```python
from build123d import *

# Parameters (mm, degrees)
SKETCH1_W           = 196.85
SKETCH1_H           = 19.05
SKETCH1_R           = 2.032
BOSS_EXTRUDE1_DEPTH = 3.175
CHAMFER1_SIZE       = 12.7
FILLET1_R           = 5.08
FILLET2_R           = 2.54
CUT_EXTRUDE1_REACH  = 100.936
FILLET3_R           = 3.175
FILLET4_R           = 0.635
FILLET5_R           = 25.4


with BuildPart() as part:
    # Sketch1 → Boss-Extrude1 (new body)
    with BuildSketch(Plane.XY):
        Rectangle(SKETCH1_W, SKETCH1_H)
        with Locations((-73.66, -5.715)):
            Circle(SKETCH1_R, mode=Mode.SUBTRACT)
        with Locations((-85.09, -5.715)):
            Circle(SKETCH1_R, mode=Mode.SUBTRACT)
        with Locations((73.66, -5.715)):
            Circle(SKETCH1_R, mode=Mode.SUBTRACT)
        with Locations((85.09, -5.715)):
            Circle(SKETCH1_R, mode=Mode.SUBTRACT)
    extrude(amount=BOSS_EXTRUDE1_DEPTH)

    # Chamfer1
    chamfer1_edges = [part.edges().sort_by_distance(p)[0] for p in [
        (-98.425, 9.525, 1.5875),
        (98.425, 9.525, 1.5875),
    ]]
    chamfer(chamfer1_edges, length=CHAMFER1_SIZE)

    # Fillet1
    fillet1_edges = [part.edges().sort_by_distance(p)[0] for p in [
        (-85.725, 9.525, 1.5875),
        (85.725, 9.525, 1.5875),
        (98.425, -3.175, 1.5875),
        (-98.425, -3.175, 1.5875),
    ]]
    fillet(fillet1_edges, radius=FILLET1_R)

    # Fillet2
    fillet2_edges = [part.edges().sort_by_distance(p)[0] for p in [
        (98.425, -9.525, 1.5875),
        (-98.425, -9.525, 1.5875),
    ]]
    fillet(fillet2_edges, radius=FILLET2_R)

    # Sketch2 → Cut-Extrude1 (cut, up to next)
    with BuildSketch(Plane.XY.offset(3.175), mode=Mode.PRIVATE) as cut_extrude1_sk1:
        Polygon((-62.264047257, 5.715), (-36.195, 1.288180654), (-10.125952743, 5.715), align=None)
    cut_extrude1_tool1 = extrude(cut_extrude1_sk1.sketch, amount=-CUT_EXTRUDE1_REACH, mode=Mode.PRIVATE) & part.part
    # Sketch2 → Cut-Extrude1 (cut, up to next)
    with BuildSketch(Plane.XY.offset(3.175), mode=Mode.PRIVATE) as cut_extrude1_sk2:
        Polygon((-69.85, 4.426819346), (-69.85, -4.426819346), (-43.780952743, 0), align=None)
    cut_extrude1_tool2 = extrude(cut_extrude1_sk2.sketch, amount=-CUT_EXTRUDE1_REACH, mode=Mode.PRIVATE) & part.part
    # Sketch2 → Cut-Extrude1 (cut, up to next)
    with BuildSketch(Plane.XY.offset(3.175), mode=Mode.PRIVATE) as cut_extrude1_sk3:
        Polygon((-36.195, -1.288180654), (-62.264047257, -5.715), (-10.125952743, -5.715), align=None)
    cut_extrude1_tool3 = extrude(cut_extrude1_sk3.sketch, amount=-CUT_EXTRUDE1_REACH, mode=Mode.PRIVATE) & part.part
    # Sketch2 → Cut-Extrude1 (cut, up to next)
    with BuildSketch(Plane.XY.offset(3.175), mode=Mode.PRIVATE) as cut_extrude1_sk4:
        Polygon((-2.54, 4.426819346), (-28.609047257, 0), (-2.54, -4.426819346), align=None)
    cut_extrude1_tool4 = extrude(cut_extrude1_sk4.sketch, amount=-CUT_EXTRUDE1_REACH, mode=Mode.PRIVATE) & part.part
    # Sketch2 → Cut-Extrude1 (cut, up to next)
    with BuildSketch(Plane.XY.offset(3.175), mode=Mode.PRIVATE) as cut_extrude1_sk5:
        Polygon((2.54, 4.426819346), (2.54, -4.426819346), (28.609047257, 0), align=None)
    cut_extrude1_tool5 = extrude(cut_extrude1_sk5.sketch, amount=-CUT_EXTRUDE1_REACH, mode=Mode.PRIVATE) & part.part
    # Sketch2 → Cut-Extrude1 (cut, up to next)
    with BuildSketch(Plane.XY.offset(3.175), mode=Mode.PRIVATE) as cut_extrude1_sk6:
        Polygon((62.264047257, 5.715), (10.125952743, 5.715), (36.195, 1.288180654), align=None)
    cut_extrude1_tool6 = extrude(cut_extrude1_sk6.sketch, amount=-CUT_EXTRUDE1_REACH, mode=Mode.PRIVATE) & part.part
    # Sketch2 → Cut-Extrude1 (cut, up to next)
    with BuildSketch(Plane.XY.offset(3.175), mode=Mode.PRIVATE) as cut_extrude1_sk7:
        Polygon((69.85, 4.426819346), (43.780952743, 0), (69.85, -4.426819346), align=None)
    cut_extrude1_tool7 = extrude(cut_extrude1_sk7.sketch, amount=-CUT_EXTRUDE1_REACH, mode=Mode.PRIVATE) & part.part
    # Sketch2 → Cut-Extrude1 (cut, up to next)
    with BuildSketch(Plane.XY.offset(3.175), mode=Mode.PRIVATE) as cut_extrude1_sk8:
        Polygon((36.195, -1.288180654), (10.125952743, -5.715), (62.264047257, -5.715), align=None)
    cut_extrude1_tool8 = extrude(cut_extrude1_sk8.sketch, amount=-CUT_EXTRUDE1_REACH, mode=Mode.PRIVATE) & part.part
    add(cut_extrude1_tool1.solids().sort_by_distance((-36.195, 4.239394, 3.175))[0], mode=Mode.SUBTRACT)
    add(cut_extrude1_tool2.solids().sort_by_distance((-61.160318, 0, 3.175))[0], mode=Mode.SUBTRACT)
    add(cut_extrude1_tool3.solids().sort_by_distance((-36.195, -4.239394, 3.175))[0], mode=Mode.SUBTRACT)
    add(cut_extrude1_tool4.solids().sort_by_distance((-11.229682, 0, 3.175))[0], mode=Mode.SUBTRACT)
    add(cut_extrude1_tool5.solids().sort_by_distance((11.229682, 0, 3.175))[0], mode=Mode.SUBTRACT)
    add(cut_extrude1_tool6.solids().sort_by_distance((36.195, 4.239394, 3.175))[0], mode=Mode.SUBTRACT)
    add(cut_extrude1_tool7.solids().sort_by_distance((61.160318, 0, 3.175))[0], mode=Mode.SUBTRACT)
    add(cut_extrude1_tool8.solids().sort_by_distance((36.195, -4.239394, 3.175))[0], mode=Mode.SUBTRACT)

    # Fillet3
    fillet3_edges = [part.edges().sort_by_distance(p)[0] for p in [
        (2.54, -4.426819346, 1.5875),
        (2.54, 4.426819346, 1.5875),
        (-2.54, 4.426819346, 1.5875),
        (-2.54, -4.426819346, 1.5875),
        (-69.85, -4.426819346, 1.5875),
        (-69.85, 4.426819346, 1.5875),
        (69.85, 4.426819346, 1.5875),
        (69.85, -4.426819346, 1.5875),
    ]]
    fillet(fillet3_edges, radius=FILLET3_R)

    # Fillet4
    fillet4_edges = [part.edges().sort_by_distance(p)[0] for p in [
        (28.609047257, 0, 1.5875),
        (-28.609047257, 0, 1.5875),
        (-43.780952743, 0, 1.5875),
        (-62.264047257, -5.715, 1.5875),
        (-10.125952743, -5.715, 1.5875),
        (62.264047257, -5.715, 1.5875),
        (10.125952743, -5.715, 1.5875),
        (10.125952743, 5.715, 1.5875),
        (62.264047257, 5.715, 1.5875),
        (43.780952743, 0, 1.5875),
        (-62.264047257, 5.715, 1.5875),
        (-10.125952743, 5.715, 1.5875),
    ]]
    fillet(fillet4_edges, radius=FILLET4_R)

    # Fillet5
    fillet5_edges = [part.edges().sort_by_distance(p)[0] for p in [
        (-36.195, -1.288180654, 1.5875),
        (36.195, -1.288180654, 1.5875),
        (36.195, 1.288180654, 1.5875),
        (-36.195, 1.288180654, 1.5875),
    ]]
    fillet(fillet5_edges, radius=FILLET5_R)


solid = part.part
```
For this review, take the finished solid that the model builds, in its own axes (mm). A direction names the side the tool comes from. Round coordinates to 2 decimals unless told otherwise and drop trailing zeros. Order: outer loops, then holes, each group sorted by start corner. A loop starts at its lowest first (then second) coordinate and runs counter-clockwise, first axis right, second up.
Q1. Mouldability with a two-part tool opening along Y and no side actions: class faces 3 (the cylindrical face through (98.05, -3.36, 1.61)), 4 (the cylindrical face through (-68.69, -3.12, 1.57)), 5 (the flat face through (-1, -9.525, 2)) as pulls with the +Y half, pulls with the -Y half, needs draft (parallel to the pull), parting line crosses it, or undercut.
Findings below:
face 3: pulls with the +Y half
face 4: undercut
face 5: pulls with the -Y half
Q2. We need section B-B, the plane z = 1.95. State how many separate pieces and enclosed holes the cut face has, plus the area to 3 significant figures.
Findings below:
separate pieces: 1
enclosed holes: 12
area: 2,680 mm2
Q3. Insertion check: P1, Ø3.5, axis at x = 73.66, y = -5.715, coming from the +Z side; P2, Ø0.7, axis at y = 0, z = 1.5, coming from the -X side; P3, Ø1.5, axis at y = 0, z = 1.5, coming from the +X side; P4, Ø0.7, axis at y = 0, z = 1.5, coming from the +X side. Each pin has a flat end and moves straight along its axis. Give the tip position at first contact, or say it passes through.
Findings below:
P1: passes through
P2: stops at x = -95.6
P3: stops at x = 96
P4: stops at x = 95.6
Q4. We need section A-A, the plane x = -73.66. Give the boundary of the cut face in (y, z) (3 decimals), plus the area to 3 significant figures.
Findings below:
outline: (-9.525, 0) - (-7.747, 0) - (-7.747, 3.175) - (-9.525, 3.175) - close; (-3.683, 0) - (9.525, 0) - (9.525, 3.175) - (-3.683, 3.175) - close
area: 47.6 mm2
Q5. We need section C-C, the plane x = 68. Give the boundary of the cut face in (y, z) (3 decimals).
Findings below:
outline: (-9.525, 0) - (-3.553, 0) - (-3.553, 3.175) - (-9.525, 3.175) - close; (3.553, 0) - (9.525, 0) - (9.525, 3.175) - (3.553, 3.175) - close
Q6. Wall thickness on line 1 (Y direction, x = -41.5, z = 2.55) (3 decimals); line 2 (Y direction, x = 39, z = 0.75) (3 decimals); line 3 (Y direction, x = -85.09, z = 2.1) (3 decimals): over which ranges is each line inside the solid? List them lowest first.
Findings below:
line 1: y = -9.525 to -5.715, -2.189 to 2.189, 5.715 to 9.525
line 2: y = -9.525 to -5.715, -1.807 to 1.807, 5.715 to 9.525
line 3: y = -9.525 to -7.747, -3.683 to 9.308
Q7. Machinability: for faces 1 (the cylindrical face through (85.54, 9.15, 1.61)), 2 (the flat face through (-15.72, -2.19, 1.61)), which of the approach directions +Z, -Z, +X, -X, +Y, -Y give a long, thin tool a straight path to every point of the face, cutting with its end or side? Answer none if there is none.
Findings below:
face 1: +Z, -Z, +X, +Y
face 2: +Z, -Z
